```python
from build123d import *

# Parameters (mm, degrees)
SKETCH3_W           = 2.25
SKETCH3_H           = 2.25
CUT_EXTRUDE1_DEPTH  = 11
CHAMFER1_SIZE       = 0.5
SKETCH4_R           = 8.5
SKETCH4_R_2         = 6
BOSS_EXTRUDE1_DEPTH = 48
SKETCH5_OUTSIDE_W   = 75.302
SKETCH5_OUTSIDE_H   = 75.302
SKETCH5_OUTSIDE_R   = 6
CUT_EXTRUDE2_DEPTH  = 18
SKETCH6_W           = 3.25
SKETCH6_H           = 3.25
CUT_EXTRUDE3_DEPTH  = 30
SKETCH7_R           = 10
SKETCH7_R_2         = 6
BOSS_EXTRUDE2_DEPTH = 2
CHAMFER2_SIZE       = 0.5


with BuildPart() as part:
    # Sketch2 → Revolve1 (revolve)
    with BuildSketch(Plane.XY, mode=Mode.PRIVATE) as revolve1_sk:
        Polygon((0, 0), (6, 0), (6, 11), (10, 11), (10, 14), (6, 14), (6, 265), (0, 265), align=None)
    revolve(revolve1_sk.sketch.rotate(Axis((0, 265, 0), (0, -1, 0)), 180), axis=Axis((0, 265, 0), (0, -1, 0)))

    # Sketch3 → Cut-Extrude1 (cut)
    with BuildSketch(Plane.XZ):
        with Locations((0, 6)):
            Rectangle(SKETCH3_W, SKETCH3_H)
    extrude(amount=-CUT_EXTRUDE1_DEPTH, mode=Mode.SUBTRACT)

    # Chamfer1
    chamfer1_edges = [part.edges().sort_by_distance(p)[0] for p in [
        (0, 0, -6),
        (6, 265, 0),
        (10, 14, 0),
        (10, 11, 0),
    ]]
    chamfer(chamfer1_edges, length=CHAMFER1_SIZE)

    # Sketch4 → Boss-Extrude1 (add)
    with BuildSketch(Plane(origin=(0, 265, 0), x_dir=(1, 0, 0), z_dir=(0, 1, 0))):
        with Locations(Location((0, 0, 0), (0, 0, 180))):
            Circle(SKETCH4_R)
        with Locations(Location((0, 0, 0), (0, 0, 180))):
            Circle(SKETCH4_R_2, mode=Mode.SUBTRACT)
    extrude(amount=-BOSS_EXTRUDE1_DEPTH)

    # Sketch5 outside → Cut-Extrude2 (cut)
    with BuildSketch(Plane(origin=(0, 265, 0), x_dir=(1, 0, 0), z_dir=(0, 1, 0))):
        Rectangle(SKETCH5_OUTSIDE_W, SKETCH5_OUTSIDE_H)
        with Locations(Location((0, 0, 0), (0, 0, 180))):
            Circle(SKETCH5_OUTSIDE_R, mode=Mode.SUBTRACT)
    extrude(amount=-CUT_EXTRUDE2_DEPTH, mode=Mode.SUBTRACT)

    # Sketch6 → Cut-Extrude3 (cut)
    with BuildSketch(Plane(origin=(0, 247, 0), x_dir=(1, 0, 0), z_dir=(0, 1, 0))):
        with Locations((0, 8.5)):
            Rectangle(SKETCH6_W, SKETCH6_H)
    extrude(amount=-CUT_EXTRUDE3_DEPTH, mode=Mode.SUBTRACT)

    # Sketch7 → Boss-Extrude2 (add)
    with BuildSketch(Plane.XZ.offset(-217)):
        with Locations(Location((0, 0, 0), (0, 0, 180))):
            Circle(SKETCH7_R)
        with Locations(Location((0, 0, 0), (0, 0, 180))):
            Circle(SKETCH7_R_2, mode=Mode.SUBTRACT)
    extrude(amount=BOSS_EXTRUDE2_DEPTH)

    # Chamfer2
    chamfer2_edges = [part.edges().sort_by_distance(p)[0] for p in [
        (10, 215, 0),
        (10, 217, 0),
        (6, 215, 0),
    ]]
    chamfer(chamfer2_edges, length=CHAMFER2_SIZE)


solid = part.part
```
Source: CAD feature listing. Evaluate the final solid. Frame: model axes, mm. A direction names the side the tool comes from. Coordinates: 2 decimals unless noted, no trailing zeros. Order: outer loops, then holes, each group sorted by start corner. A loop starts at its lowest first (then second) coordinate and runs counter-clockwise, first axis right, second up. Notation, with made-up numbers: M 16.5,-35.75 L 39.5,-35.75 A9 ccw 39.5,-29.75 Z; hole C 19.5,-32 d6. An arc over 180 degrees is marked long. Write each question's results on one line, items separated by ' | '. Start each with the question number.
1) Contact query for flat-ended pins moving along their axis: pin 1 Ø2 at (x, z) = (-6, 5.5) entering from -Y; pin 2 Ø1.6 at (x, y) = (0.5, 225.5) entering from -Z (3 decimals); pin 3 Ø12 at (x, y) = (-2, 88.5) entering from -Z. Output: stop coordinate, or through.
2) Section query A-A (y = 49). Return the cut outline in (x, z), plus the area to 3 significant figures.
3) Draft query along Y for faces 6 (the face through (0, 6, -6)), 7 (the face through (-6, 247, 2)), 8 (the face through (-4, 215, 6)), 9 (the face through (-5.723, 115.654, -1.802)). Return one class per face: released by +Y, released by -Y, zero draft, split by the parting line, or undercut.
4) Line query: line 1 (Y direction, x = 8, z = 0.25); line 2 (Y direction, x = 8.5, z = 2.25); line 3 (Z direction, x = 0.75, y = 243) (3 decimals). Output: solid intervals per line, ascending. Write a range as from..to.
5) Access query for faces 1 (the face through (10, 13, 0)), 2 (the face through (0, 265, 0)), 3 (the face through (0.1, 14, 6.2)), 4 (the face through (0, 11, 6)), 5 (the face through (-0.351, 232.21, 8.493)). Directions: +Z, -Z, +X, -X, +Y, -Y. A direction counts if a zero-diameter tool reaches every point of the face in a straight line with its end or side. Return the directions, or none.
Answers:
1) pin 1: stops at y = 11 | pin 2: stops at z = -6.875 | pin 3: stops at z = -6
2) outline: C 0,0 d12 | area: 113 mm^2
3) face 6: zero draft | face 7: released by +Y | face 8: undercut | face 9: undercut
4) line 1: y = 11..14, 215..247 | line 2: y = 11..14, 215..217 | line 3: z = -6.875..8.467
5) face 1: +Y, -Y | face 2: +Z, -Z, +X, -X, +Y | face 3: none | face 4: -Y | face 5: +Y
